Read the model definition and answer for the solid it produces. Units are mm, in the model's axes. A direction names the side the tool comes from. Coordinates: 2 decimals unless noted, no trailing zeros. Loops run counter-clockwise (first coordinate to the right, second up) from the corner with the lowest first, then second, coordinate; pieces in that order, holes last. Notation, with made-up numbers: (89.5, 58.5) - (148.5, 58.5) arc R21 cw to (148.5, 93.5) - close; hole circle Ø4 at (-3, -9.75). An arc over 180 degrees is marked (long way). Use CSV: the item, a comma, the result in double quotes.
```python
from build123d import *

# Parameters (mm, degrees)
SCHIZZO1_W                   = 12
SCHIZZO1_H                   = 12
ESTRUSIONE_ESTRUSIONE1_DEPTH = 56.75
RACCORDO1_R                  = 2
ESTRUSIONE_ESTRUSIONE3_START = -8.75
SCHIZZO3_W                   = 8
SCHIZZO3_H                   = 10
SCHIZZO3_W_2                 = 10
SCHIZZO3_H_2                 = 8
ESTRUSIONE_ESTRUSIONE3_DEPTH = 96
FORO_FILETTATO_M2_5_3_D      = 2.05
FORO_FILETTATO_M2_5_3_DEPTH  = 6.884117865
FORO_FILETTATO_M2_5_3_TIP    = 0.615882135
FORO_FILETTATO_M2_5_4_D      = 2.05
FORO_FILETTATO_M2_5_4_DEPTH  = 6.884117865
FORO_FILETTATO_M2_5_4_TIP    = 0.615882135


with BuildPart() as part:
    # Schizzo1 → Estrusione-Estrusione1 (new, symmetric)
    with BuildSketch(Plane.XY):
        Rectangle(SCHIZZO1_W, SCHIZZO1_H)
    extrude(amount=ESTRUSIONE_ESTRUSIONE1_DEPTH, both=True)

    # Raccordo1
    raccordo1_edges = [part.edges().sort_by_distance(p)[0] for p in [
        (-6, 0, 56.75),
        (0, -6, 56.75),
        (6, 0, 56.75),
        (0, -6, -56.75),
        (-6, 0, -56.75),
        (0, 6, -56.75),
        (6, 0, -56.75),
        (-6, 6, 0),
        (0, 6, 56.75),
    ]]
    fillet(raccordo1_edges, radius=RACCORDO1_R)

    # Schizzo3 → Estrusione-Estrusione3 (add)
    with BuildSketch(Plane.XY.offset(56.75).offset(ESTRUSIONE_ESTRUSIONE3_START)):
        with Locations((0, 11)):
            Rectangle(SCHIZZO3_W, SCHIZZO3_H)
        with Locations((-11, 0)):
            Rectangle(SCHIZZO3_W_2, SCHIZZO3_H_2)
    extrude(amount=-ESTRUSIONE_ESTRUSIONE3_DEPTH)

    # Schizzo5 → Foro filettato M2.5-1 (revolve, cut)
    with BuildSketch(Plane(origin=(1, 11, 48), x_dir=(0, -1, 0), z_dir=(1, 0, 0))):
        Polygon((0, 0), (0, 7.5), (1.025, 6.884117865), (1.025, 0), align=None)
    foro_filettato_m2_5_1 = revolve(axis=Axis((1, 11, 54.35), (0, 0, -1)), mode=Mode.SUBTRACT)

    # Schizzo8 → Foro filettato M2.5-2 (revolve, cut)
    with BuildSketch(Plane(origin=(-11, -1, 48), x_dir=(0, -1, 0), z_dir=(1, 0, 0))):
        Polygon((0, 0), (0, 7.5), (1.025, 6.884117865), (1.025, 0), align=None)
    foro_filettato_m2_5_2 = revolve(axis=Axis((-11, -1, 54.35), (0, 0, -1)), mode=Mode.SUBTRACT)

    # Specchia2: Foro filettato M2.5-1, Foro filettato M2.5-2 across plane
    add(foro_filettato_m2_5_1.mirror(Plane.XY), mode=Mode.SUBTRACT)
    add(foro_filettato_m2_5_2.mirror(Plane.XY), mode=Mode.SUBTRACT)

    # Foro filettato M2.5-3
    with Locations(Plane(origin=(4, 0, 0), x_dir=(0, 0, -1), z_dir=(1, 0, 0))):
        with Locations((-25, 10), (25, 10)):
            Hole(FORO_FILETTATO_M2_5_3_D / 2, depth=FORO_FILETTATO_M2_5_3_DEPTH)
            with Locations((0, 0, -(FORO_FILETTATO_M2_5_3_DEPTH + FORO_FILETTATO_M2_5_3_TIP / 2))):  # 118° drill point
                Cone(0, FORO_FILETTATO_M2_5_3_D / 2, FORO_FILETTATO_M2_5_3_TIP, mode=Mode.SUBTRACT)

    # Foro filettato M2.5-4
    with Locations(Plane(origin=(0, -4, 0), x_dir=(-1, 0, 0), z_dir=(0, -1, 0))):
        with Locations((10, 25), (10, -25)):
            Hole(FORO_FILETTATO_M2_5_4_D / 2, depth=FORO_FILETTATO_M2_5_4_DEPTH)
            with Locations((0, 0, -(FORO_FILETTATO_M2_5_4_DEPTH + FORO_FILETTATO_M2_5_4_TIP / 2))):  # 118° drill point
                Cone(0, FORO_FILETTATO_M2_5_4_D / 2, FORO_FILETTATO_M2_5_4_TIP, mode=Mode.SUBTRACT)


solid = part.part
```
Q1. The part is cut by section A-A on z = -32. Determine the outline of the cut face in (x, y).
Reported:
outline,"(-16, -4) - (-6, -4) - (-6, -6) - (6, -6) - (6, 6) - (4, 6) - (4, 16) - (-4, 16) - (-4, 6) arc R2 ccw to (-6, 4) - (-16, 4) - close"
Q2. Find the intervals of material crossed by probe 1 along Z at (x, y) = (-10, 0) (3 decimals); probe 2 along Y at (x, z) = (-1, 25) (3 decimals); probe 3 along X at (y, z) = (-1, -43) (3 decimals), in increasing order. Write a range as [from, to].
Reported:
probe 1,"z = [-48, -26.025], [-23.975, 23.975], [26.025, 48]"
probe 2,"y = [-6, 8.975], [11.025, 16]"
probe 3,"x = [-16, -12.025], [-9.975, 6]"
Q3. A tool of negligible diameter and unlimited length cuts with its end or side. For faces 1 (the face through (0.955, 12.024, -44.606)), 2 (the face through (4, 11, 1)), 3 (the face through (-1, 11, -48)), from which of +Z, -Z, +X, -X, +Y, -Y can it reach the whole face along a straight path? Write none if from no direction.
Reported:
face 1,"-Z"
face 2,"+Z, -Z, +X, +Y"
face 3,"-Z, +X, -X, +Y"
Q4. Given P1, Ø2.5, axis at x = -12.5, y = -0.5, coming from the -Z side; P2, Ø5, axis at x = -9.5, z = -16.5, coming from the -Y side; P3, Ø1.8, axis at x = -10, z = -25, coming from the +Y side, each flat-ended and moving along its own axis, determine where each tip first touches the part or whether it passes through.
Reported:
P1,"stops at z = -48"
P2,"stops at y = -4"
P3,"stops at y = 4"
Q5. For a pull along X with two mould halves and no side action, classify faces 4 (the face through (-5.43, 5.4, -0.77)), 5 (the face through (-10.133, -0.51, 23.984)), 6 (the face through (0.08, -5.4, -56.18)) as +X half, -X half, draft (parallel to the pull), parting line (faces both ways), or undercut.
Reported:
face 4,"-X half"
face 5,"undercut"
face 6,"draft"
